For this review, take the finished solid that the model builds, in its own axes (mm). Face numbers are marked on the shaded views. A direction names the side the tool comes from. Give positions to 0.01 mm unless a question says otherwise; leave off trailing zeros. Write each loop counter-clockwise with the first axis right and the second up, starting at its lowest first coordinate (ties: lowest second). Pieces come first, ordered by that corner, then holes. Notation, with made-up numbers: M -19,56 L -5,56 A30 cw -5,88 Z; hole C -10,4 d2. An arc over 180 degrees is marked long. Answer as a JSON object with one key per item and string values. Group by question number.
```python
from build123d import *

# Parameters (mm, degrees)
SKETCH1_R           = 34
SKETCH1_R_2         = 25
BOSS_EXTRUDE1_DEPTH = 51.5
BOSS_EXTRUDE2_REACH = 87.5
SKETCH2_R           = 34
SKETCH2_R_2         = 25


with BuildPart() as part:
    # Sketch1 → Boss-Extrude1 (new body, symmetric)
    with BuildSketch(Plane(origin=(0, 0, 0), x_dir=(1, 0, 0), z_dir=(0, 1, 0))):
        Circle(SKETCH1_R)
        Circle(SKETCH1_R_2, mode=Mode.SUBTRACT)
    extrude(amount=BOSS_EXTRUDE1_DEPTH, both=True)

    # Sketch2 → Boss-Extrude2 (add, up to next)
    with BuildSketch(Plane(origin=(51.5, 0, 0), x_dir=(0, 0, -1), z_dir=(1, 0, 0)), mode=Mode.PRIVATE) as boss_extrude2_sk1:
        Circle(SKETCH2_R)
        Circle(SKETCH2_R_2, mode=Mode.SUBTRACT)
    boss_extrude2_tool1 = extrude(boss_extrude2_sk1.sketch, amount=-BOSS_EXTRUDE2_REACH, mode=Mode.PRIVATE) - part.part
    add(boss_extrude2_tool1.solids().sort_by_distance((51.5, 0, 33.038335))[0])


solid = part.part
```
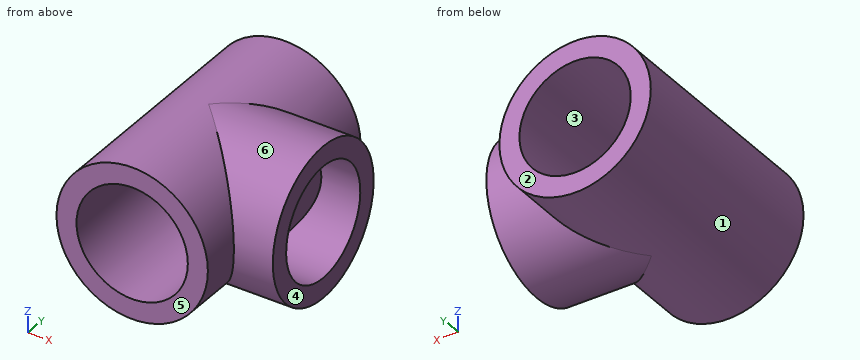
Item 1: Consider section A-A (z = 0). Give the boundary of the cut face in (x, y).
Item 2: Draft analysis for pull direction X (two halves, no side actions). For the marked faces 1, 2, 3 and 4, state which applies: released by +X, released by -X, zero draft, split by the parting line, or undercut.
Item 3: To check wall thickness, follow probe 1 along X at (y, z) = (24.5, -1); probe 2 along Z at (x, y) = (27, 10); probe 3 along Y at (x, z) = (34, -6.5). State the ranges of each line that lie inside material, in increasing order.
Item 4: Insertion check: P1, Ø1.5, axis at x = -1.5, y = -38, coming from the +Z side; P2, Ø10, axis at x = 14, y = -31, coming from the -Z side; P3, Ø12, axis at x = -20, y = -35.5, coming from the -Z side. Each pin has a flat end and moves straight along its axis. Give the tip position at first contact, or say it passes through.
Item 5: Machinability: for the marked faces 5 and 6, which of the approach directions +Z, -Z, +X, -X, +Y, -Y give a long, thin tool a straight path to every point of the face, cutting with its end or side? Answer none if there is none.
Item 6: Consider section D-D (x = 43.5). Give the boundary of the cut face in (y, z).
Item 7: Consider section B-B (y = 0). Give the boundary of the cut face in (x, z), plus the area to 3 significant figures.
Item 8: Consider section C-C (x = -9.5). Give the boundary of the cut face in (y, z).
Result set:
{
 "1": {"outline": "M -34,-51.5 L -25,-51.5 L -25,51.5 L -34,51.5 Z; M 25,-51.5 L 34,-51.5 L 34,-34 L 51.5,-34 L 51.5,-25 L 34,-25 L 34,25 L 51.5,25 L 51.5,34 L 34,34 L 34,51.5 L 25,51.5 Z"},
 "2": {"face 1": "split by the parting line", "face 2": "zero draft", "face 3": "undercut", "face 4": "released by +X"},
 "3": {"probe 1": "x = -33.99 to -24.98, 24.98 to 33.99", "probe 2": "z = -32.5 to -22.91, -20.66 to 20.66, 22.91 to 32.5", "probe 3": "y = -33.37 to -24.14, 24.14 to 33.37"},
 "4": {"P1": "stops at z = 33.99", "P2": "stops at z = -32.79", "P3": "stops at z = -30.98"},
 "5": {"face 5": "+Z, -Z, +X, -X, -Y", "face 6": "+X"},
 "6": {"outline": "C 0,0 d68; hole C 0,0 d50"},
 "7": {"outline": "M 0,-34 L 51.5,-34 L 51.5,-25 L 23.04,-25 A34 ccw 23.04,25 L 51.5,25 L 51.5,34 L 0,34 A34 ccw Z; hole C 0,0 d50", "area": "2,310 mm^2"},
 "8": {"outline": "M -51.5,-32.65 L 51.5,-32.65 L 51.5,-23.12 L -51.5,-23.12 Z; M -51.5,23.12 L 51.5,23.12 L 51.5,32.65 L -51.5,32.65 Z"}
}
